Source: CAD feature listing. Evaluate the final solid. Frame: model axes, mm. Coordinates: 2 decimals unless noted, no trailing zeros. Write each loop counter-clockwise with the first axis right and the second up, starting at its lowest first coordinate (ties: lowest second). Pieces come first, ordered by that corner, then holes. Notation, with made-up numbers: (57.25, -7) - (112.25, -7) arc R24 cw to (112.25, 27) - close; hole circle Ø8 at (60.5, -22). An arc over 180 degrees is marked (long way). One line per question, with ' | ' between items. Start each with the question number.
Q1. Line query: line 1 (Z direction, x = 1.45, y = 7.25); line 2 (Z direction, x = 1.75, y = -4.75); line 3 (Z direction, x = 1.55, y = 0.25). Output: solid intervals per line, ascending.
Q2. Cut plane B-B, the plane y = -12. Return loops of the section in (x, z) (3 decimals).
Q3. Cut plane C-C, the plane x = 0.6. Give the number of separate pieces and of enclosed holes in the cut face, plus the area to 3 significant figures.
Q4. Cut plane D-D, the plane z = 29. Return loops of the section in (x, y), plus the area to 3 significant figures.
Q5. Contact query for flat-ended pins moving along their axis: P1, Ø1.5, axis at x = 2, z = -30, coming from the +Y side; P2, Ø0.6, axis at x = 1.5, y = -2.5, coming from the -Z side; P3, Ø1, axis at x = 1, z = 47.5, coming from the -Y side. Output: stop coordinate, or through.
Q6. Cut plane A-A, the plane y = -0.5. Return loops of the section in (x, z), plus the area to 3 significant figures.
Autodesk Inventor part; units mm, degrees
ref_plane "YZ Plane" through (0, 0, 0) normal (1, 0, 0) x (0, 1, 0)
ref_plane "XZ Plane" through (0, 0, 0) normal (0, 1, 0) x (-1, 0, 0)
ref_plane "XY Plane" through (0, 0, 0) normal (0, 0, 1) x (1, 0, 0)
sketch "Sketch2" plane through (0, 0, 0) normal (1, 0, 0) x (0, 1, 0)
  line L0 (14, -51) -> (11, -51)
  line L1 (-14, 51) -> (-11, 51)
  line L2 (14, 51) -> (14, 48)
  line L3 (-14, 51) -> (-14, 48)
  line L4 (14, -48) -> (11, -48)
  line L5 (11, -51) -> (11, -48)
  line L6 (0, -71.4) -> (0, 71.4) construction
  line L7 (3.975, -51) -> (3.975, -48)
  line L8 (-3.975, -51) -> (-3.975, -48)
  line L9 (1.5, -48) -> (1.5, -46)
  line L10 (1.5, -46) -> (2.65, -46)
  line L11 (2.65, -46) -> (2.65, -43.6)
  line L12 (2.65, -43.6) -> (1.5, -43.6)
  line L13 (1.5, -43.6) -> (1.5, -43)
  line L14 (1.5, -43) -> (-1.5, -43)
  line L15 (-1.5, -43) -> (-1.5, -43.6)
  line L16 (-1.5, -43.6) -> (-2.65, -43.6)
  line L17 (-2.65, -43.6) -> (-2.65, -46)
  line L18 (-2.65, -46) -> (-1.5, -46)
  line L19 (-1.5, -46) -> (-1.5, -48)
  line L20 (11, -51) -> (-14, -51)
  line L21 (1.5, -48) -> (-14, -48)
  line L22 (3.975, -48) -> (1.5, -48)
  line L23 (11, -48) -> (3.975, -48)
  line L24 (-23.2, 0) -> (41.2, 0) construction
  line L25 (-11, -51) -> (-11, -48)
  line L26 (14, 48) -> (11, 48)
  line L27 (11, 51) -> (11, 48)
  line L28 (3.975, 51) -> (3.975, 48)
  line L29 (-3.975, 51) -> (-3.975, 48)
  line L30 (1.5, 48) -> (1.5, 46)
  line L31 (1.5, 46) -> (2.65, 46)
  line L32 (2.65, 46) -> (2.65, 43.6)
  line L33 (2.65, 43.6) -> (1.5, 43.6)
  line L34 (1.5, 43.6) -> (1.5, 43)
  line L35 (1.5, 43) -> (-1.5, 43)
  line L36 (-1.5, 43) -> (-1.5, 43.6)
  line L37 (-1.5, 43.6) -> (-2.65, 43.6)
  line L38 (-2.65, 43.6) -> (-2.65, 46)
  line L39 (-2.65, 46) -> (-1.5, 46)
  line L40 (-1.5, 46) -> (-1.5, 48)
  line L41 (1.5, 48) -> (-14, 48)
  line L42 (3.975, 48) -> (1.5, 48)
  line L43 (11, 48) -> (3.975, 48)
  line L44 (-11, 51) -> (-11, 48)
  line L45 (3.975, 51) -> (11, 51)
  line L46 (-3.975, 51) -> (3.975, 51)
  line L47 (11, -48) -> (11, -1.5)
  line L48 (-11, 48) -> (-11, 18)
  line L49 (14, 21) -> (11, 21) construction
  line L50 (14, -21) -> (11, -21) construction
  line L51 (14, 18) -> (11, 18)
  line L52 (14, -18) -> (11, -18)
  line L53 (14, -3.975) -> (11, -3.975)
  line L54 (14, 3.975) -> (11, 3.975)
  line L55 (11, 1.5) -> (9, 1.5)
  line L56 (9, 1.5) -> (9, 2.65)
  line L57 (9, 2.65) -> (6.6, 2.65)
  line L58 (6.6, 2.65) -> (6.6, 1.5)
  line L59 (6.6, 1.5) -> (6, 1.5)
  line L60 (6, 1.5) -> (6, -1.5)
  line L61 (6, -1.5) -> (6.6, -1.5)
  line L62 (6.6, -1.5) -> (6.6, -2.65)
  line L63 (6.6, -2.65) -> (9, -2.65)
  line L64 (9, -2.65) -> (9, -1.5)
  line L65 (11, -1.5) -> (9, -1.5)
  line L66 (14, -3.975) -> (14, -18)
  line L67 (14, 3.975) -> (14, -3.975)
  line L68 (11, 1.5) -> (11, 48)
  line L69 (11, -1.5) -> (11, 1.5)
  line L70 (-14, 18) -> (-11, 18)
  line L71 (-14, -18) -> (-11, -18)
  line L72 (-14, -3.975) -> (-11, -3.975)
  line L73 (-14, 3.975) -> (-11, 3.975)
  line L74 (-11, 1.5) -> (-9, 1.5)
  line L75 (-9, 1.5) -> (-9, 2.65)
  line L76 (-9, 2.65) -> (-6.6, 2.65)
  line L77 (-6.6, 2.65) -> (-6.6, 1.5)
  line L78 (-6.6, 1.5) -> (-6, 1.5)
  line L79 (-6, 1.5) -> (-6, -1.5)
  line L80 (-6, -1.5) -> (-6.6, -1.5)
  line L81 (-6.6, -1.5) -> (-6.6, -2.65)
  line L82 (-6.6, -2.65) -> (-9, -2.65)
  line L83 (-9, -2.65) -> (-9, -1.5)
  line L84 (-11, -1.5) -> (-9, -1.5)
  line L85 (-14, 3.975) -> (-14, -3.975)
  line L86 (-14, -3.975) -> (-14, -18)
  line L87 (-14, 18) -> (-14, 3.975)
  line L88 (-14, -18) -> (-14, -51)
  line L89 (14, -18) -> (14, -51)
  line L90 (14, 18) -> (14, 3.975)
  line L91 (-11, -3.975) -> (-11, -18)
  line L92 (-11, -18) -> (-11, -48)
  line L93 (-11, 18) -> (-11, 3.975)
  line L94 (14, 48) -> (14, 18)
  line L95 (-14, 48) -> (-14, 18)
  line L96 (-11, 51) -> (-3.975, 51)
  line L97 (11, 51) -> (14, 51)
  line L98 (-11, 3.975) -> (-11, 1.5)
  line L99 (-11, 1.5) -> (-11, -1.5)
  line L100 (-11, -1.5) -> (-11, -3.975)
  line L101 (8, -34.5052) -> (8, -37.5052)
  line L102 (-8, -37.5052) -> (8, -37.5052)
  line L103 (-8, -34.5052) -> (-8, -37.5052)
  line L104 (8, -34.5052) -> (-8, -34.5052)
  line L105 (8, -24) -> (-8, -24)
  line L106 (-8, -24) -> (-8, -21)
  line L107 (8, -21) -> (-8, -21)
  line L108 (8, -24) -> (8, -21)
  line L109 (32, 21) -> (17, 21)
  line L110 (17, 21) -> (17, 24)
  line L111 (32, 24) -> (17, 24)
  line L112 (32, 21) -> (32, 24)
  line L113 (8, 21) -> (-8, 21)
  line L114 (-8, 21) -> (-8, 24)
  line L115 (8, 24) -> (-8, 24)
  line L116 (8, 21) -> (8, 24)
  line L117 (-8, 34.4948) -> (-8, 37.4948)
  line L118 (8, 37.4948) -> (-8, 37.4948)
  line L119 (8, 34.4948) -> (8, 37.4948)
  line L120 (-8, 34.4948) -> (8, 34.4948)
  point P0 (0, 0)
  dimension "d5" = 3
  dimension "d6" = 3
  dimension "d8" = 2.4
  dimension "d9" = 5.3
  dimension "d10" = 3
  dimension "d11" = 2
  dimension "d12" = 5
  dimension "d13" = 7.95
  dimension "d14" = 28
  dimension "d15" = 102
  dimension "d17" = 42
  dimension "d18" = 3
  dimension "d19" = 3
  dimension "d20" = 2
  dimension "d21" = 5
  dimension "d22" = 2.4
  dimension "d23" = 5.3
  dimension "d24" = 3
  dimension "d25" = 7.95
extrude "Extrusion1" add sketch "Sketch2" along normal blind 3 contours L20 L7 L23 L5 | L23 L22 L9 L10 L11 L12 L13 L14 L15 L16 L17 L18 L19 L21 L92 L91 L100 L84 L83 L82 L81 L80 L79 L78 L77 L76 L75 L74 L98 L93 L48 L41 L40 L39 L38 L37 L36 L35 L34 L33 L32 L31 L30 L42 L43 L68 L55 L56 L57 L58 L59 L60 L61 L62 L63 L64 L65 L47 | L52 L47 L53 L66 | L20 L25 L21 L8 | L54 L68 L51 L90 | L71 L86 L72 L91 | L43 L28 L45 L27 | L87 L70 L93 L73 | L29 L41 L44 L96
equation "\"d13\" = 1.5 * d9"
equation "\"d25\" = 1.5 * d23"
properties part number "Bearing-Side"
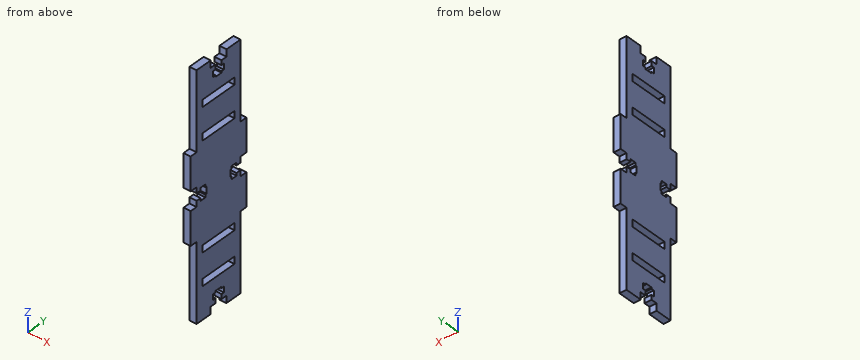
Reply:
1) line 1: z = -51 to -37.51, -34.51 to -24, -21 to -2.65, 2.65 to 21, 24 to 34.49, 37.49 to 51 | line 2: z = -51 to -37.51, -34.51 to -24, -21 to 21, 24 to 34.49, 37.49 to 51 | line 3: z = -43 to -37.51, -34.51 to -24, -21 to 21, 24 to 34.49, 37.49 to 43
2) outline: (0, -18) - (3, -18) - (3, -3.975) - (0, -3.975) - close; (0, 3.975) - (3, 3.975) - (3, 18) - (0, 18) - close
3) separate pieces: 1 | enclosed holes: 4 | area: 2,090 mm^2
4) outline: (0, -11) - (3, -11) - (3, 11) - (0, 11) - close | area: 66.0 mm^2
5) P1: stops at y = 11 | P2: stops at z = -48 | P3: stops at y = -11
6) outline: (0, -43) - (3, -43) - (3, -37.51) - (0, -37.51) - close; (0, -34.51) - (3, -34.51) - (3, -24) - (0, -24) - close; (0, -21) - (3, -21) - (3, 21) - (0, 21) - close; (0, 24) - (3, 24) - (3, 34.49) - (0, 34.49) - close; (0, 37.49) - (3, 37.49) - (3, 43) - (0, 43) - close | area: 222 mm^2
